For this review, use the dimensioned drawing (mm, ordinates from the lowest corner) and the shaded views. A direction names the side the tool comes from. Coordinates: 2 decimals unless noted, no trailing zeros. Loops run counter-clockwise (first coordinate to the right, second up) from the corner with the lowest first, then second, coordinate; pieces in that order, holes last. Notation, with made-up numbers: (38.25, 76) -> (60.25, 76) arc R27 cw to (60.25, 114) -> close; hole circle Ø9 at (7, 30.25). An arc over 180 degrees is marked (long way). Answer as a JSON object with one key per item and string values.
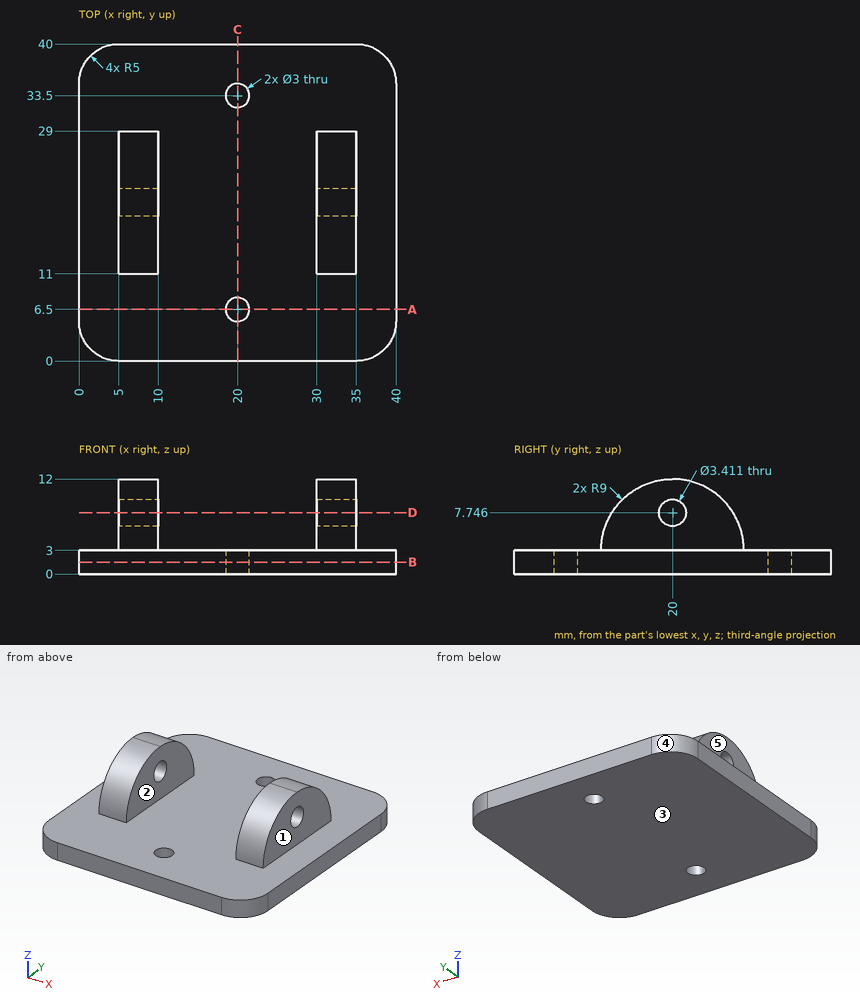
1) Add section A-A, the plane y = 6.5. Give the boundary of the cut face in (x, z).
Completed:
{"outline": "(0, 0) -> (18.5, 0) -> (18.5, 3) -> (0, 3) -> close; (21.5, 0) -> (40, 0) -> (40, 3) -> (21.5, 3) -> close"}
2) Add section C-C, the plane x = 20. Give the boundary of the cut face in (y, z).
Completed:
{"outline": "(0, 0) -> (5, 0) -> (5, 3) -> (0, 3) -> close; (8, 0) -> (32, 0) -> (32, 3) -> (8, 3) -> close; (35, 0) -> (40, 0) -> (40, 3) -> (35, 3) -> close"}
3) Add section D-D, the plane z = 7.75. Give the boundary of the cut face in (x, y) (1 decimal).
Completed:
{"outline": "(5, 12.4) -> (10, 12.4) -> (10, 18.3) -> (5, 18.3) -> close; (5, 21.7) -> (10, 21.7) -> (10, 27.6) -> (5, 27.6) -> close; (30, 12.4) -> (35, 12.4) -> (35, 18.3) -> (30, 18.3) -> close; (30, 21.7) -> (35, 21.7) -> (35, 27.6) -> (30, 27.6) -> close"}
4) For the marked faces 1, 2, 3, 4 and 5, list the 3-axis set-ups (+Z, -Z, +X, -X, +Y, -Y) from which the entire face can be reached by the end or side of a thin tool; tool diameter is ignored.
Completed:
{"face 1": "+Z, +X, +Y, -Y", "face 2": "+Z, +Y, -Y", "face 3": "-Z, +X, -X, +Y, -Y", "face 4": "+Z, -Z, -X, +Y", "face 5": "+Z, -X, +Y, -Y"}
5) Wall thickness on probe 1 along Y at (x, z) = (20, 1.7); probe 2 along X at (y, z) = (28, 6.5); probe 3 along Z at (x, y) = (19, 20): over which ranges is each line inside the solid? List them lowest first.
Completed:
{"probe 1": "0 to 5, 8 to 32, 35 to 40", "probe 2": "5 to 10, 30 to 35", "probe 3": "0 to 3"}
6) Clearance check with flat-ended pins moving along their axes: pin 1 Ø5 at (x, y) = (7.5, 32) entering from +Z; pin 2 Ø2.5 at (y, z) = (16.5, 9) entering from -X; pin 3 Ø2.5 at (x, y) = (20, 33.5) entering from -Z; pin 4 Ø4.5 at (y, z) = (23.5, 7) entering from +X. State where each tip first meets the part, or that it passes through.
Completed:
{"pin 1": "z = 3", "pin 2": "x = 5", "pin 3": "through", "pin 4": "x = 35"}
7) Add section B-B, the plane z = 1.5. Give the boundary of the cut face in (x, y).
Completed:
{"outline": "(0, 5) arc R5 ccw to (5, 0) -> (35, 0) arc R5 ccw to (40, 5) -> (40, 35) arc R5 ccw to (35, 40) -> (5, 40) arc R5 ccw to (0, 35) -> close; hole circle Ø3 at (20, 6.5); hole circle Ø3 at (20, 33.5)"}
